The figure shows three views and two pictorial views of one solid part (mm, origin at its lowest corner). Answer the questions. A direction names the side the tool comes from. Coordinates: 2 decimals unless noted, no trailing zeros. Order: outer loops, then holes, each group sorted by start corner. A loop starts at its lowest first (then second) coordinate and runs counter-clockwise, first axis right, second up. Notation, with made-up numbers: (18, -1.5) - (49, -1.5) arc R28 ccw to (49, 23.5) - close; hole circle Ø11 at (79, 3). An arc over 180 degrees is marked (long way). Answer as a JSON object with one key per item and string values. Group by question number.
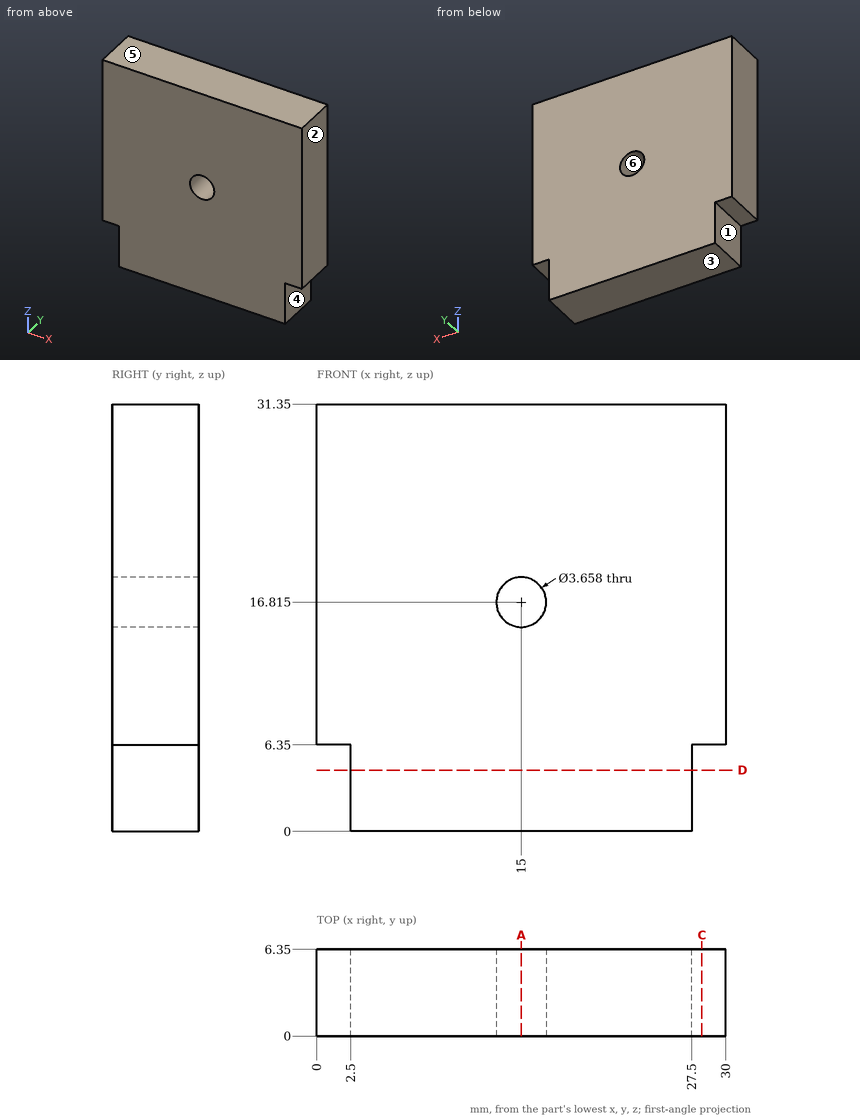
1. Straight lines are drawn through the part: L1, parallel to Z at x = 15.75, y = 3.75; L2, parallel to X at y = 5.5, z = 5. For each, find the intervals that lie inside material, in ascending order.
2. For a pull along Z with two mould halves and no side action, classify the marked faces 3, 4, 5 and 6 as pulls with the +Z half, pulls with the -Z half, needs draft (parallel to the pull), parting line crosses it, or undercut.
3. For the marked faces 1 and 2, determine the directions among +Z, -Z, +X, -X, +Y, -Y from which every point of the face is accessible in a straight line to the end or side of a thin tool.
4. Given pin 1 (1.9 mm diameter, centred on y = 2.5, z = 2, fed in from -X); pin 2 (1.2 mm diameter, centred on x = 28.5, y = 2, fed in from -Z); pin 3 (1 mm diameter, centred on y = 5, z = 13, fed in from -X), each flat-ended and moving along its own axis, determine where each tip first touches the part or whether it passes through.
5. A cutting plane is placed at C-C on x = 28.25. Write down the section's boundary in (y, z).
6. A cutting plane is placed at D-D on z = 4.5. Write down the section's boundary in (x, y).
7. A cutting plane is placed at A-A on x = 15. Write down the section's boundary in (y, z), and give its area (3 significant figures).
Derived:
{
 "1": {"L1": "z = 0 to 15.15, 18.48 to 31.35", "L2": "x = 2.5 to 27.5"},
 "2": {"face 3": "pulls with the -Z half", "face 4": "needs draft", "face 5": "pulls with the +Z half", "face 6": "undercut"},
 "3": {"face 1": "-Z, -X, +Y, -Y", "face 2": "+Z, -Z, +X, +Y, -Y"},
 "4": {"pin 1": "stops at x = 2.5", "pin 2": "stops at z = 6.35", "pin 3": "stops at x = 0"},
 "5": {"outline": "(0, 6.35) - (6.35, 6.35) - (6.35, 31.35) - (0, 31.35) - close"},
 "6": {"outline": "(2.5, 0) - (27.5, 0) - (27.5, 6.35) - (2.5, 6.35) - close"},
 "7": {"outline": "(0, 0) - (6.35, 0) - (6.35, 14.99) - (0, 14.99) - close; (0, 18.64) - (6.35, 18.64) - (6.35, 31.35) - (0, 31.35) - close", "area": "176 mm2"}
}
